Autodesk Inventor part; units mm, degrees
ref_plane "Work Plane1" through (0, 0, 10) normal (0, 0, 1) x (1, 0, 0)
ref_plane "YZ Plane" through (0, 0, 0) normal (1, 0, 0) x (0, 1, 0)
ref_plane "XZ Plane" through (0, 0, 0) normal (0, 1, 0) x (-1, 0, 0)
ref_plane "Work Plane1" through (0, 0, 10) normal (0, 0, 1) x (1, 0, 0)
sketch "Sketch1" plane through (0, 0, 10) normal (0, 0, 1) x (1, 0, 0)
  line L0 (-4.0299, -0.3538) -> (-2.2322, 1.4439) construction
  arc A0 (-1.4439, 2.2322) -> (-2.2322, 1.4439) centre (-0.9299, 0.9299) ccw construction
  line L1 (-1.4439, 2.2322) -> (0.3538, 4.0299) construction
  line L2 (-37.8299, 42.8299) -> (-37.8299, 37.8299) construction
  line L3 (-37.8299, 37.8299) -> (-42.9208, 37.8299) construction
  line L4 (-37.8299, 42.2137) -> (-37.8299, 45.8299) construction
  line L5 (-37.8299, 45.8299) -> (-4.0299, 45.8299) construction
  line L6 (-4.0299, 45.8299) -> (-4.0299, 42.2137) construction
  line L7 (-4.0299, 4.0299) -> (0.3538, 4.0299)
  circle A1 centre (-20.9299, 20.9299) radius 17.5
  line L8 (-20.9299, 58.9723) -> (17.1124, 20.9299) construction
  line L9 (17.1124, 20.9299) -> (-20.9299, -17.1124) construction
  line L10 (-20.9299, -17.1124) -> (-58.9723, 20.9299) construction
  line L11 (-58.9723, 20.9299) -> (-20.9299, 58.9723) construction
  line L12 (-20.9299, 58.9723) -> (-20.9299, -17.1124) construction
  line L13 (17.1124, 20.9299) -> (-58.9723, 20.9299) construction
  line L14 (-20.9299, 58.9723) -> (32.8701, 58.9723) construction
  line L15 (-43.4299, 43.4299) -> (1.5701, 43.4299) construction
  line L16 (1.5701, 43.4299) -> (1.5701, -1.5701) construction
  line L17 (1.5701, -1.5701) -> (-43.4299, -1.5701) construction
  line L18 (-43.4299, -1.5701) -> (-43.4299, 43.4299) construction
  line L19 (-43.4299, 43.4299) -> (1.5701, -1.5701) construction
  line L20 (1.5701, 43.4299) -> (-43.4299, -1.5701) construction
  line L21 (-43.4299, 5.3876) -> (-43.4299, 36.4723)
  line L22 (-43.4299, 36.4723) -> (-36.4723, 43.4299)
  line L23 (-36.4723, 43.4299) -> (-5.3876, 43.4299)
  line L24 (-5.3876, 43.4299) -> (1.5701, 36.4723)
  line L25 (1.5701, 36.4723) -> (1.5701, 5.3876)
  line L26 (1.5701, 5.3876) -> (-5.3876, -1.5701)
  line L27 (-5.3876, -1.5701) -> (-36.4723, -1.5701)
  line L28 (-36.4723, -1.5701) -> (-43.4299, 5.3876)
  line L29 (-4.0299, 42.2137) -> (-37.8299, 42.2137)
  line L30 (-4.0299, -0.3538) -> (-4.0299, 4.0299)
  circle A2 centre (-20.9299, 20.9299) radius 1.5
  line L31 (-10.9299, 10.9299) -> (-30.9299, 10.9299) construction
  line L32 (-30.9299, 10.9299) -> (-30.9299, 30.9299) construction
  line L33 (-30.9299, 30.9299) -> (-10.9299, 30.9299) construction
  line L34 (-10.9299, 30.9299) -> (-10.9299, 10.9299) construction
  line L35 (-10.9299, 10.9299) -> (-30.9299, 30.9299) construction
  line L36 (-30.9299, 10.9299) -> (-10.9299, 30.9299) construction
  circle A3 centre (-30.9299, 30.9299) radius 1.4
  circle A4 centre (-30.9299, 10.9299) radius 1.4
  circle A5 centre (-10.9299, 10.9299) radius 1.4
  line L37 (-45.8299, 37.8299) -> (-42.0723, 37.8299) construction
  line L38 (-42.1723, 37.7299) -> (-45.8299, 37.7299)
  line L39 (-45.8299, 37.7299) -> (-45.8299, 4.1299)
  line L40 (-45.8299, 4.1299) -> (-42.1723, 4.1299)
  line L41 (-42.1723, 4.1299) -> (-42.1723, 37.7299)
  line L42 (-45.8299, 4.0299) -> (-42.0723, 4.0299) construction
  line L43 (-45.8299, 37.8299) -> (-42.0723, 37.8299)
  line L44 (-37.7299, 45.8299) -> (-4.1299, 45.8299)
  line L45 (-4.1299, 45.8299) -> (-4.1299, 42.1723)
  line L46 (-4.1299, 42.1723) -> (-37.7299, 42.1723)
  line L47 (-37.7299, 42.1723) -> (-37.7299, 45.8299)
  line L48 (0.4701, 37.8299) -> (0.4701, 4.0299) construction
  line L49 (0.4701, 4.0299) -> (3.9701, 4.0299) construction
  line L50 (3.9701, 37.8299) -> (3.9701, 4.0299) construction
  line L51 (0.4701, 37.8299) -> (3.9701, 37.8299) construction
  line L52 (-45.8299, -3.9701) -> (-4.0299, -3.9701) construction
  line L53 (0.3124, 37.7299) -> (3.9701, 37.7299)
  line L54 (3.9701, 37.7299) -> (3.9701, 4.1299)
  line L55 (3.9701, 4.1299) -> (0.3124, 4.1299)
  line L56 (0.3124, 4.1299) -> (0.3124, 37.7299)
  line L57 (-4.1713, -0.3538) -> (-37.7299, -0.3538)
  line L58 (-37.7299, -0.3538) -> (-37.7299, -3.9701)
  line L59 (-37.7299, -3.9701) -> (-4.1713, -3.9701)
  line L60 (-4.1713, -3.9701) -> (-4.1713, -0.3538)
  point P0 (-37.8299, 4.0299)
  dimension "d18" = 53.8
  dimension "d19" = 45
  dimension "d20" = 53.8
  dimension "d21" = 45
  dimension "d22" = 45
  dimension "d30" = 20
  dimension "d31" = 20
  dimension "d32" = 2.8
  dimension "d33" = 2.8
  dimension "d34" = 2.8
  dimension "d35" = 3
  dimension "d36" = 0.1
  dimension "d37" = 0.1
  dimension "d38" = 0.1
  dimension "d39" = 0.1
extrude "Extrusion1" add sketch "Sketch1" along normal blind 8 contours L30 L26 L57 L28 L41 L22 L46 L24 L56 L7 | L7 L26 L30 | L56 L24 L25 L26 | L26 L25 L24 L53 L54 L55 | L60 L59 L58 L57 L28 L27 L26 | L26 L27 L28 L57 | L46 L22 L29 L24 | L24 L29 L45 | L40 L39 L38 L22 L21 L28 | L28 L21 L22 L41 | L29 L22 L23 L24 | L24 L23 L22 L29 L47 L44 L45 | L47 L29 L22 | A1 | A2 | A3 | A4 | A5
sketch "Skizze4" plane through (0, 0, 18) normal (0, 0, 1) x (1, 0, 0)
  line L0 (-37.7299, 42.1723) -> (-42.1723, 37.7299)
  line L1 (-42.1723, 37.7299) -> (-45.8299, 37.7299)
  line L2 (-45.8299, 37.7299) -> (-45.8299, 4.1299) construction
  line L3 (-45.8299, 4.1299) -> (-42.1723, 4.1299)
  line L4 (-42.1723, 4.1299) -> (-37.6885, -0.3538)
  line L5 (-37.6885, -0.3538) -> (-37.7299, -0.3538)
  line L6 (-37.7299, -0.3538) -> (-37.7299, -3.9701)
  line L7 (-37.7299, -3.9701) -> (-4.1713, -3.9701) construction
  line L8 (-4.1713, -3.9701) -> (-4.1713, -0.3538)
  line L9 (-4.1713, -0.3538) -> (0.3124, 4.1299)
  line L10 (0.3124, 4.1299) -> (3.9701, 4.1299)
  line L11 (3.9701, 4.1299) -> (3.9701, 37.7299) construction
  line L12 (3.9701, 37.7299) -> (0.3124, 37.7299)
  line L13 (0.3124, 37.7299) -> (-4.1299, 42.1723)
  line L14 (-4.1299, 42.1723) -> (-4.1299, 45.8299)
  line L15 (-4.1299, 45.8299) -> (-37.7299, 45.8299) construction
  line L16 (-37.7299, 45.8299) -> (-37.7299, 42.1723)
  line L17 (-37.9299, 46.0299) -> (-3.9299, 46.0299) construction
  line L18 (-3.9299, 46.0299) -> (-3.9299, 42.2551)
  line L19 (-3.9299, 42.2551) -> (0.3953, 37.9299)
  line L20 (0.3953, 37.9299) -> (4.1701, 37.9299)
  line L21 (4.1701, 37.9299) -> (4.1701, 3.9299) construction
  line L22 (4.1701, 3.9299) -> (0.3953, 3.9299)
  line L23 (0.3953, 3.9299) -> (-3.9713, -0.4367)
  line L24 (-3.9713, -0.4367) -> (-3.9713, -4.1701)
  line L25 (-3.9713, -4.1701) -> (-37.9299, -4.1701) construction
  line L26 (-37.9299, -4.1701) -> (-37.9299, -0.3953)
  line L27 (-37.9299, -0.3953) -> (-42.2551, 3.9299)
  line L28 (-42.2551, 3.9299) -> (-46.0299, 3.9299)
  line L29 (-46.0299, 3.9299) -> (-46.0299, 37.9299) construction
  line L30 (-46.0299, 37.9299) -> (-42.2551, 37.9299)
  line L31 (-42.2551, 37.9299) -> (-37.9299, 42.2551)
  line L32 (-37.9299, 42.2551) -> (-37.9299, 46.0299)
  line L33 (-45.8299, 37.7299) -> (-45.8299, 37.9299)
  line L34 (-4.1299, 45.8299) -> (-37.7299, 45.8299)
  line L35 (-37.7299, 45.8299) -> (-37.9299, 45.8299)
  line L36 (-4.1299, 45.8299) -> (-3.9299, 45.8299)
  line L37 (3.9701, 37.7299) -> (3.9701, 37.9299)
  line L38 (3.9701, 4.1299) -> (3.9701, 37.7299)
  line L39 (3.9701, 4.1299) -> (3.9701, 3.9299)
  line L40 (-4.1713, -3.9701) -> (-3.9713, -3.9701)
  line L41 (-37.7299, -3.9701) -> (-37.9299, -3.9701)
  line L42 (-45.8299, 4.1299) -> (-45.8299, 3.9299)
  point P0 (0, 0)
  dimension "d40" = 0.2
extrude "IM_offset" add sketch "Skizze4" against normal up to surface (8 mm away)
sketch "Sketch20" plane through (0, 0, 18) normal (0, 0, 1) x (1, 0, 0)
  line L0 (-3.9299, 45.8299) -> (-37.9299, 45.8299)
  line L1 (-37.9299, 45.8299) -> (-37.9299, 42.2551)
  line L2 (-37.9299, 42.2551) -> (-42.2551, 37.9299)
  line L3 (-42.2551, 37.9299) -> (-45.8299, 37.9299)
  line L4 (-45.8299, 37.9299) -> (-45.8299, 3.9299)
  line L5 (-42.2551, 3.9299) -> (-45.8299, 3.9299)
  line L6 (-37.9299, -0.3953) -> (-42.2551, 3.9299)
  line L7 (-37.9299, -3.9701) -> (-37.9299, -0.3953)
  line L8 (-3.9713, -3.9701) -> (-37.9299, -3.9701)
  line L9 (-3.9713, -3.9701) -> (-3.9713, -0.4367)
  line L10 (-3.9713, -0.4367) -> (0.3953, 3.9299)
  line L11 (0.3953, 3.9299) -> (3.9701, 3.9299)
  line L12 (3.9701, 3.9299) -> (3.9701, 37.9299)
  line L13 (3.9701, 37.9299) -> (0.3953, 37.9299)
  line L14 (0.3953, 37.9299) -> (-3.9299, 42.2551)
  line L15 (-3.9299, 42.2551) -> (-3.9299, 45.8299)
  circle A0 centre (-20.9299, 20.9299) radius 11.5
  line L16 (-12.9299, 28.9299) -> (-28.9299, 12.9299) construction
  line L17 (-28.9299, 28.9299) -> (-12.9299, 12.9299) construction
  point P0 (0, 0)
  dimension "d113" = 23
  dimension "d115" = 16
  dimension "d116" = 16
extrude "Extrusion18" cut sketch "Sketch20" against normal through all contours A0
properties part number "20_Cube_Insert_Eyepiece"
Work out the finished part from the listing and answer in its coordinate system (mm). A direction names the side the tool comes from. Give positions to 0.01 mm unless a question says otherwise; leave off trailing zeros. Write each loop counter-clockwise with the first axis right and the second up, starting at its lowest first coordinate (ties: lowest second). Pieces come first, ordered by that corner, then holes.
(1) The part is cut by section A-A on y = 31. Write down the section's boundary in (x, z), plus the area to 3 significant figures.
Final values:
outline: (-45.83, 10) - (-26.48, 10) - (-26.48, 18) - (-45.83, 18) - close; (-15.38, 10) - (3.97, 10) - (3.97, 18) - (-15.38, 18) - close
area: 310 mm2
(2) The part is cut by section D-D on y = 1. Write down the section's boundary in (x, z).
Final values:
outline: (-39.33, 10) - (-2.53, 10) - (-2.53, 18) - (-39.33, 18) - close
(3) The part is cut by section B-B on x = -31. Write down the section's boundary in (y, z), plus the area to 3 significant figures.
Final values:
outline: (-3.97, 10) - (15.38, 10) - (15.38, 18) - (-3.97, 18) - close; (26.48, 10) - (45.83, 10) - (45.83, 18) - (26.48, 18) - close
area: 310 mm2
(4) The mould has two halves that part along X. Classify faces 5 (the flat face through (-37.93, -2, 14)), 6 (the cylindrical face through (-23.4, 9.7, 14.1)), 7 (the flat face through (2, 37.93, 14)): pulls with the +X half, pulls with the -X half, needs draft (parallel to the pull), parting line crosses it, or undercut.
Final values:
face 5: pulls with the -X half
face 6: undercut
face 7: needs draft
(5) Which of the six approach directions +Z, -Z, +X, -X, +Y, -Y give full straight-line access (tool end or side, diameter ignored) to faces 1 (the flat face through (-44, 3.93, 14)), 2 (the flat face through (-37.93, 44, 14)), 3 (the flat face through (-3.971, -2, 14)), 4 (the flat face through (-3.93, 44, 14))?
Final values:
face 1: +Z, -Z, -X, -Y
face 2: +Z, -Z, -X, +Y
face 3: +Z, -Z, +X, -Y
face 4: +Z, -Z, +X, +Y
(6) Flat-ended cylindrical pins translate along their axes: pin 1 Ø4 at (x, z) = (-43.5, 13.5) entering from -Y; pin 2 Ø1.1 at (x, z) = (-45, 13.5) entering from +Y; pin 3 Ø3 at (y, z) = (43, 13.5) entering from -X (3 decimals). Find the tip coordinate at first contact, or state that the pin passes through.
Final values:
pin 1: stops at y = 3.17
pin 2: stops at y = 37.93
pin 3: stops at x = -38.685
(7) The part is cut by section C-C on z = 13. Write down the section's boundary in (x, y).
Final values:
outline: (-45.83, 3.93) - (-42.26, 3.93) - (-37.93, -0.4) - (-37.93, -3.97) - (-3.97, -3.97) - (-3.97, -0.44) - (0.4, 3.93) - (3.97, 3.93) - (3.97, 37.93) - (0.4, 37.93) - (-3.93, 42.26) - (-3.93, 45.83) - (-37.93, 45.83) - (-37.93, 42.26) - (-42.26, 37.93) - (-45.83, 37.93) - close; hole circle Ø23 at (-20.93, 20.93)
(8) Straight lines are drawn through the part: line 1 (X direction, y = 29.5, z = 15); line 2 (X direction, y = 14, z = 15.75); line 3 (X direction, y = -2, z = 16). For each, find the intervals that lie inside material, in ascending order.
Final values:
line 1: x = -45.83 to -28.6, -13.26 to 3.97
line 2: x = -45.83 to -30.11, -11.75 to 3.97
line 3: x = -37.93 to -3.97
